The figure shows three views and two pictorial views of one solid part (mm, origin at its lowest corner). Answer the questions. A direction names the side the tool comes from. Round coordinates to 2 decimals unless told otherwise and drop trailing zeros. Order: outer loops, then holes, each group sorted by start corner. A loop starts at its lowest first (then second) coordinate and runs counter-clockwise, first axis right, second up. Notation, with made-up numbers: (-1, -0.5) -> (51, -0.5) arc R16 cw to (51, 23.5) -> close; hole circle Ø1 at (26, 11.5). An arc over 180 degrees is marked (long way). One line per item, written item: value. Start each with the question number.
1. Consider line 1 (X direction, y = 19, z = 24); line 2 (X direction, y = 35, z = 17.5). Determine where each line is inside the solid, lowest interval first.
2. The mould has two halves that part along Y. Classify the marked faces 1, 2, 3 and 4: released by +Y, released by -Y, zero draft, split by the parting line, or undercut.
3. For the marked faces 5 and 6, determine the directions among +Z, -Z, +X, -X, +Y, -Y from which every point of the face is accessible in a straight line to the end or side of a thin tool.
4. Flat-ended cylindrical pins translate along their axes: pin 1 Ø2 at (y, z) = (21.5, 5) entering from -X; pin 2 Ø12 at (x, y) = (109.5, 16) entering from -Z. Find the tip coordinate at first contact, or state that the pin passes through.
5. Section D-D (x = 23) is taken. Give the vertices of the cut face in (y, z), then the cut area to 3 significant figures.
6. Section C-C (z = 28) is taken. Give the vertices of the cut face in (x, y).
7. Section A-A (x = 101.5) is taken. Give the vertices of the cut face in (y, z), then the cut area to 3 significant figures.
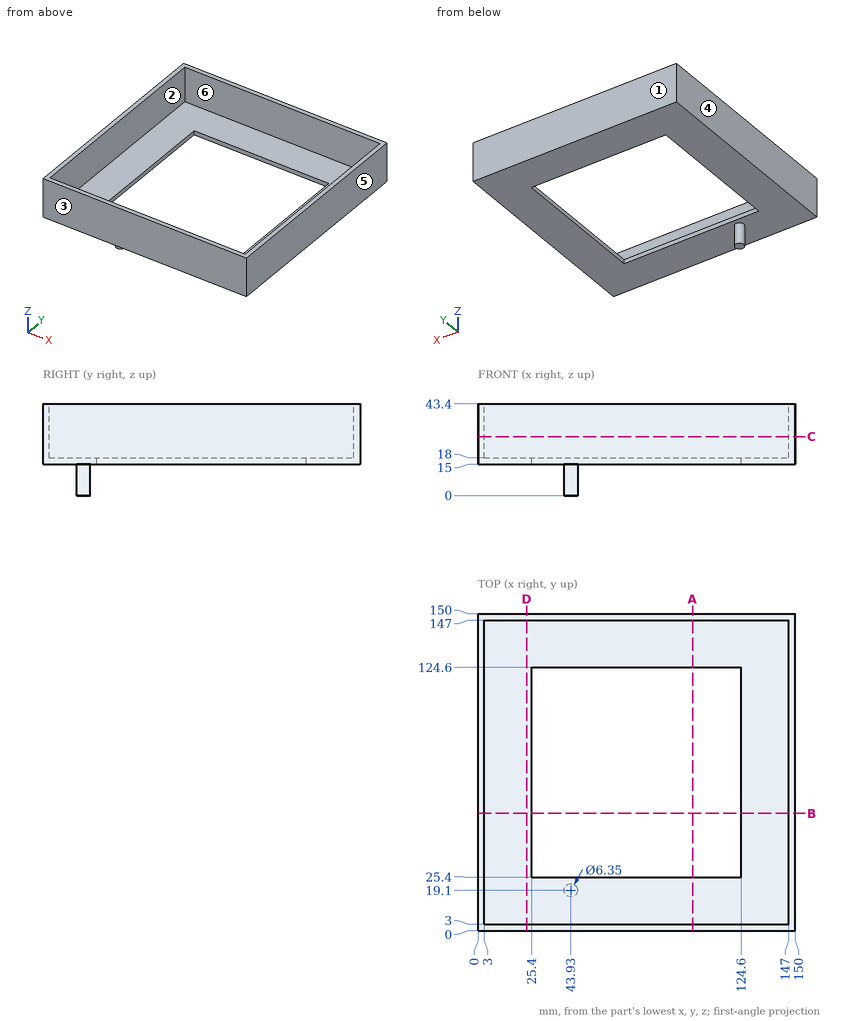
Answer:
1. line 1: 0 to 3, 147 to 150
1. line 2: 0 to 25.4, 124.6 to 150
2. face 1: released by +Y
2. face 2: undercut
2. face 3: released by -Y
2. face 4: zero draft
3. face 5: +Z, -Z, +X, +Y, -Y
3. face 6: +Z
4. pin 1: x = 41.08
4. pin 2: z = 15
5. outline: (0, 15) -> (150, 15) -> (150, 43.4) -> (147, 43.4) -> (147, 18) -> (3, 18) -> (3, 43.4) -> (0, 43.4) -> close
5. area: 602 mm^2
6. outline: (0, 0) -> (150, 0) -> (150, 150) -> (0, 150) -> close; hole (3, 3) -> (147, 3) -> (147, 147) -> (3, 147) -> close
7. outline: (0, 15) -> (25.4, 15) -> (25.4, 18) -> (3, 18) -> (3, 43.4) -> (0, 43.4) -> close; (124.6, 15) -> (150, 15) -> (150, 43.4) -> (147, 43.4) -> (147, 18) -> (124.6, 18) -> close
7. area: 305 mm^2
